The listing builds one solid part. Answer for the finished solid, in the listing's coordinates (mm). A direction names the side the tool comes from. Give positions to 0.01 mm unless a question says otherwise; leave off trailing zeros. Order: outer loops, then holes, each group sorted by start corner. A loop starts at its lowest first (then second) coordinate and runs counter-clockwise, first axis right, second up. Notation, with made-up numbers: (37, -28.5) - (95, -28.5) arc R5 cw to (95, -19.5) - close; hole circle Ø7 at (64, 36). An arc over 180 degrees is marked (long way). Answer as a JSON object with one key per item and string values. Group by question number.
Q1. A cutting plane is placed at B-B, the plane x = -33. Give the vertices of the cut face in (y, z), and give its area (3 significant figures).
Q2. A cutting plane is placed at D-D, the plane z = 17.5. Give the vertices of the cut face in (x, y).
Q3. A cutting plane is placed at A-A, the plane z = 6.35. Give the vertices of the cut face in (x, y), and give its area (3 significant figures).
Q4. The mould has two halves that part along Z. Classify faces 4 (the face through (-25.65, 39.21, 16.53)), 5 (the face through (-46, -7, 0)), 6 (the face through (-22.73, 37, 13)): released by +Z, released by -Z, zero draft, split by the parting line, or undercut.
Q5. Consider line 1 (Y direction, x = -24.45, z = 6.35); line 2 (Y direction, x = -27.2, z = 19.05); line 3 (Y direction, x = -42, z = 2.75). Determine where each line is inside the solid, lowest interval first.
Q6. Given pin 1 (12 mm diameter, centred on y = 42, z = 16.5, fed in from -X); pin 2 (4 mm diameter, centred on x = -31, z = 3.5, fed in from -Y); pin 3 (7.5 mm diameter, centred on y = 41.14, z = 6.35, fed in from +X); pin 4 (1.5 mm diameter, centred on x = -37, z = 11.5, fed in from +Y), each flat-ended and moving along its own axis, determine where each tip first touches the part or whether it passes through.
Q7. A cutting plane is placed at C-C, the plane y = 39. Give the vertices of the cut face in (x, z), and give its area (3 significant figures).
Q8. For faces 1 (the face through (-28.493, 41, 13)), 2 (the face through (-28.493, -41, 13)), 3 (the face through (-46, -7, 25.4)), determine the directions among +Z, -Z, +X, -X, +Y, -Y from which every point of the face is accessible in a straight line to the end or side of a thin tool.
Autodesk Inventor part; units mm, degrees
ref_plane "YZ Plane" through (0, 0, 0) normal (1, 0, 0) x (0, 1, 0)
ref_plane "XZ Plane" through (0, 0, 0) normal (0, 1, 0) x (-1, 0, 0)
ref_plane "XY Plane" through (0, 0, 0) normal (0, 0, 1) x (1, 0, 0)
sketch "Sketch1" plane through (0, 0, 0) normal (0, 0, 1) x (1, 0, 0)
  arc A0 (-11.3451, -36.1483) -> (17.6265, -10) centre (-17.6849, 0) ccw
  line L0 (17.6265, -10) -> (19.0151, -10)
  line L1 (19.0151, -10) -> (19.0151, 10)
  line L2 (19.0151, 10) -> (17.6265, 10)
  arc A1 (17.6265, 10) -> (-11.3451, 36.1483) centre (-17.6849, 0) ccw
  line L3 (-11.3451, 36.1483) -> (-11.3451, 46.225)
  line L4 (-17.6951, 46.225) -> (-11.3451, 46.225)
  line L5 (-17.6951, 25.4) -> (-17.6951, 46.225)
  arc A2 (-17.6951, -25.4) -> (-17.6951, 25.4) centre (-17.6849, 0) ccw
  line L6 (-17.6951, -46.225) -> (-17.6951, -25.4)
  line L7 (-17.6951, -46.225) -> (-11.3451, -46.225)
  line L8 (-11.3451, -36.1483) -> (-11.3451, -46.225)
  circle A3 centre (-17.6849, 0) radius 25.4
  arc A4 (-22.7296, 27.4808) -> (-22.7296, -27.4808) centre (-17.6849, 0) ccw
  line L9 (-22.7296, -46.5279) -> (-22.7296, -27.4808)
  line L10 (-22.7296, -46.5279) -> (-28.4927, -46.5279)
  line L11 (-22.7296, -27.4808) -> (-22.7296, 27.4808) construction
  arc A5 (-28.4927, 35.7486) -> (-28.4927, -35.7486) centre (-17.6849, 0) ccw
  line L12 (-22.7296, 27.4808) -> (-22.7296, 37.0044)
  line L13 (-28.4927, -46.5279) -> (-28.4927, -35.7486)
  line L14 (-17.6849, 0) -> (-81.3039, 0) construction
  line L15 (-22.7296, 46.5279) -> (-22.7296, 27.4808)
  line L16 (-22.7296, 46.5279) -> (-28.4927, 46.5279)
  line L17 (-28.4927, 46.5279) -> (-28.4927, 35.7486)
  point P0 (0, 0)
  dimension "d0" = 2.54
  dimension "d1" = 0
  dimension "d2" = 0.3029
extrude "Extrusion1" add sketch "Sketch1" along normal blind 25.4 contours A4 L9 L10 L13 A5 L17 L16 L15 L12
sketch "Sketch2" plane through (-28.4927, 35.7486, 0) normal (-1, 0, 0) x (0, 0, 1)
  line L0 (0, -8.2678) -> (0, 10.7793)
  line L1 (25.4, 10.7793) -> (25.4, 0)
  line L2 (0, 10.7793) -> (25.4, 0) construction
  line L3 (12.7, 5.3897) -> (0, 5.3897) construction
  line L4 (12.7, 5.3897) -> (25.4, 5.3897) construction
  circle A0 centre (19.05, 5.3897) radius 3.175
  circle A1 centre (6.35, 5.3897) radius 3.175
  point P0 (0, -35.7486)
  dimension "d5" = 6.35
extrude "Extrusion2" cut sketch "Sketch2" against normal blind 25.4
ref_plane "Work Plane1" through (-28.4927, 0, 0) normal (0, 1, 0) x (1, 0, 0)
mirror "Mirror1" about plane through (-28.4927, 0, 0) normal (0, 1, 0) of "Extrusion2"
properties part number "dremelClamp"
Reply:
{
 "1": {"outline": "(-34.06, 0) - (-23.37, 0) - (-23.37, 25.4) - (-34.06, 25.4) - close; (23.37, 0) - (34.06, 0) - (34.06, 25.4) - (23.37, 25.4) - close", "area": "543 mm^2"},
 "2": {"outline": "(-28.49, -46.53) - (-22.73, -46.53) - (-22.73, -43.91) - (-28.49, -43.91) - close; (-28.49, -38.37) - (-22.73, -38.37) - (-22.73, -27.48) arc R27.94 cw to (-22.73, 27.48) - (-22.73, 38.37) - (-28.49, 38.37) - (-28.49, 35.75) arc R37.35 ccw to (-28.49, -35.75) - close; (-28.49, 43.91) - (-22.73, 43.91) - (-22.73, 46.53) - (-28.49, 46.53) - close"},
 "3": {"outline": "(-28.49, -46.53) - (-22.73, -46.53) - (-22.73, -44.31) - (-28.49, -44.31) - close; (-28.49, -37.96) - (-22.73, -37.96) - (-22.73, -27.48) arc R27.94 cw to (-22.73, 27.48) - (-22.73, 37.96) - (-28.49, 37.96) - (-28.49, 35.75) arc R37.35 ccw to (-28.49, -35.75) - close; (-28.49, 44.31) - (-22.73, 44.31) - (-22.73, 46.53) - (-28.49, 46.53) - close", "area": "912 mm^2"},
 "4": {"face 4": "undercut", "face 5": "released by -Z", "face 6": "zero draft"},
 "5": {"line 1": "y = -46.53 to -44.31, -37.96 to -27.11, 27.11 to 37.96, 44.31 to 46.53", "line 2": "y = -46.53 to -44.31, -37.96 to -26.27, 26.27 to 37.96, 44.31 to 46.53", "line 3": "y = -28.35 to -13.76, 13.76 to 28.35"},
 "6": {"pin 1": "stops at x = -28.49", "pin 2": "stops at y = -35.59", "pin 3": "stops at x = -22.73", "pin 4": "stops at y = 32.41"},
 "7": {"outline": "(-28.49, 0) - (-22.73, 0) - (-22.73, 4) - (-28.49, 4) - close; (-28.49, 8.7) - (-22.73, 8.7) - (-22.73, 16.7) - (-28.49, 16.7) - close; (-28.49, 21.4) - (-22.73, 21.4) - (-22.73, 25.4) - (-28.49, 25.4) - close", "area": "92.3 mm^2"},
 "8": {"face 1": "+Z, -Z, -X, +Y", "face 2": "+Z, -Z, -X, -Y", "face 3": "+Z, +X, -X, +Y, -Y"}
}
